Source: CAD feature listing. Evaluate the final solid. Frame: model axes, mm. A direction names the side the tool comes from. Round coordinates to 2 decimals unless told otherwise and drop trailing zeros.
from build123d import *

# Parameters (mm, degrees)
ESQUISSE1_R             = 7
BOSS_EXTRU_1_DEPTH      = 10
BOSS_EXTRU_2_START      = -4
ESQUISSE2_R             = 7
ESQUISSE2_R_2           = 2.5
BOSS_EXTRU_2_DEPTH      = 4
ESQUISSE3_R             = 3.375
ENL_V_MAT_EXTRU_1_DEPTH = 261.780079761
ESQUISSE4_R             = 3.375
ENL_V_MAT_EXTRU_2_DEPTH = 261.780079761


with BuildPart() as part:
    # Esquisse1 → Boss.-Extru.1 (new body)
    with BuildSketch(Plane.XY):
        with BuildLine():
            Line((-250, 17.5), (250, 17.5))
            ThreePointArc((250, 17.5), (257.071067812, 14.571067812), (260, 7.5))
            Line((260, 7.5), (260, -7.5))
            ThreePointArc((260, -7.5), (257.071067812, -14.571067812), (250, -17.5))
            Line((250, -17.5), (-250, -17.5))
            ThreePointArc((-250, -17.5), (-257.071067812, -14.571067812), (-260, -7.5))
            Line((-260, -7.5), (-260, 7.5))
            ThreePointArc((-260, 7.5), (-257.071067812, 14.571067812), (-250, 17.5))
        make_face()
        with Locations((-240, 0)):
            Circle(ESQUISSE1_R, mode=Mode.SUBTRACT)
        with Locations((-180, 0)):
            Circle(ESQUISSE1_R, mode=Mode.SUBTRACT)
        with Locations((-120, 0)):
            Circle(ESQUISSE1_R, mode=Mode.SUBTRACT)
        with Locations((-60, 0)):
            Circle(ESQUISSE1_R, mode=Mode.SUBTRACT)
        Circle(ESQUISSE1_R, mode=Mode.SUBTRACT)
        with Locations((60, 0)):
            Circle(ESQUISSE1_R, mode=Mode.SUBTRACT)
        with Locations((120, 0)):
            Circle(ESQUISSE1_R, mode=Mode.SUBTRACT)
        with Locations((180, 0)):
            Circle(ESQUISSE1_R, mode=Mode.SUBTRACT)
        with Locations((240, 0)):
            Circle(ESQUISSE1_R, mode=Mode.SUBTRACT)
    extrude(amount=BOSS_EXTRU_1_DEPTH)

    # Esquisse2 → Boss.-Extru.2 (add)
    # profile 1 of 9: a face of its own
    with BuildSketch(Plane.XY.offset(10).offset(BOSS_EXTRU_2_START)):
        with Locations((-240, 0)):
            Circle(ESQUISSE2_R)
        with Locations((-240, 0)):
            Circle(ESQUISSE2_R_2, mode=Mode.SUBTRACT)
    # profile 2 of 9: a face of its own
    with BuildSketch(Plane.XY.offset(10).offset(BOSS_EXTRU_2_START)):
        with Locations((-180, 0)):
            Circle(ESQUISSE2_R)
        with Locations((-180, 0)):
            Circle(ESQUISSE2_R_2, mode=Mode.SUBTRACT)
    # profile 3 of 9: a face of its own
    with BuildSketch(Plane.XY.offset(10).offset(BOSS_EXTRU_2_START)):
        with Locations((-120, 0)):
            Circle(ESQUISSE2_R)
        with Locations((-120, 0)):
            Circle(ESQUISSE2_R_2, mode=Mode.SUBTRACT)
    # profile 4 of 9: a face of its own
    with BuildSketch(Plane.XY.offset(10).offset(BOSS_EXTRU_2_START)):
        with Locations((-60, 0)):
            Circle(ESQUISSE2_R)
        with Locations((-60, 0)):
            Circle(ESQUISSE2_R_2, mode=Mode.SUBTRACT)
    # profile 5 of 9: a face of its own
    with BuildSketch(Plane.XY.offset(10).offset(BOSS_EXTRU_2_START)):
        Circle(ESQUISSE2_R)
        Circle(ESQUISSE2_R_2, mode=Mode.SUBTRACT)
    # profile 6 of 9: a face of its own
    with BuildSketch(Plane.XY.offset(10).offset(BOSS_EXTRU_2_START)):
        with Locations((60, 0)):
            Circle(ESQUISSE2_R)
        with Locations((60, 0)):
            Circle(ESQUISSE2_R_2, mode=Mode.SUBTRACT)
    # profile 7 of 9: a face of its own
    with BuildSketch(Plane.XY.offset(10).offset(BOSS_EXTRU_2_START)):
        with Locations((120, 0)):
            Circle(ESQUISSE2_R)
        with Locations((120, 0)):
            Circle(ESQUISSE2_R_2, mode=Mode.SUBTRACT)
    # profile 8 of 9: a face of its own
    with BuildSketch(Plane.XY.offset(10).offset(BOSS_EXTRU_2_START)):
        with Locations((180, 0)):
            Circle(ESQUISSE2_R)
        with Locations((180, 0)):
            Circle(ESQUISSE2_R_2, mode=Mode.SUBTRACT)
    # profile 9 of 9: a face of its own
    with BuildSketch(Plane.XY.offset(10).offset(BOSS_EXTRU_2_START)):
        with Locations((240, 0)):
            Circle(ESQUISSE2_R)
        with Locations((240, 0)):
            Circle(ESQUISSE2_R_2, mode=Mode.SUBTRACT)
    extrude(amount=BOSS_EXTRU_2_DEPTH)

    # Esquisse3 → Enlèv. mat.-Extru.1 (cut, through all)
    with BuildSketch(Plane.XY.offset(10)):
        with Locations((20.000000156, -12.000000313)):
            Circle(ESQUISSE3_R)
    extrude(amount=-ENL_V_MAT_EXTRU_1_DEPTH, mode=Mode.SUBTRACT)

    # Esquisse4 → Enlèv. mat.-Extru.2 (cut, through all)
    with BuildSketch(Plane.XY.offset(10)):
        with Locations((240.000000156, -12.000000313)):
            Circle(ESQUISSE4_R)
    extrude(amount=-ENL_V_MAT_EXTRU_2_DEPTH, mode=Mode.SUBTRACT)


solid = part.part
1) Pull-direction query (X, two-part tool) for faces 1 (the face through (-256.99, -14.65, 4.93)), 2 (the face through (-177, 0, 6)), 3 (the face through (257.15, -14.49, 4.93)); classes: released by +X, released by -X, zero draft, split by the parting line, or undercut.
Taken from the geometry:
face 1: released by -X
face 2: undercut
face 3: released by +X
2) Material intervals for line 1 (Y direction, x = -180, z = 9); line 2 (X direction, y = -12, z = 2.25) (3 decimals); line 3 (X direction, y = -9.5, z = 1.5), sorted ascending.
Taken from the geometry:
line 1: y = -17.5 to -2.5, 2.5 to 17.5
line 2: x = -258.93 to 16.625, 23.375 to 236.625, 243.375 to 258.93
line 3: x = -259.8 to 17.73, 22.27 to 237.73, 242.27 to 259.8
3) Section query A-A on z = 8.5. State how many separate pieces and enclosed holes the cut face has, then the cut area to 3 significant figures.
Taken from the geometry:
separate pieces: 1
enclosed holes: 11
area: 17,900 mm2
4) Contact query for flat-ended pins moving along their axis: P1, Ø1.5, axis at y = -8.5, z = 9, coming from the -X side; P2, Ø11, axis at x = 120, y = 0.5, coming from the -Z side; P3, Ø3, axis at y = -14, z = 2.5, coming from the -X side. Output: stop coordinate, or through.
Taken from the geometry:
P1: stops at x = -260
P2: stops at z = 6
P3: stops at x = -258.66
5) Reachability of faces 4 (the face through (4, 8, 0)), 5 (the face through (6.466, -2.681, 2.958)) from +Z, -Z, +X, -X, +Y, -Y: full face, straight path, thin tool, end or side. Return the list, or none.
Taken from the geometry:
face 4: -Z, +X, -X, +Y, -Y
face 5: -Z
